Geometry: final body of the model. Coordinates: model frame, mm. Face numbers are marked on the shaded views. A direction names the side the tool comes from. Coordinates: 2 decimals unless noted, no trailing zeros. Write each loop counter-clockwise with the first axis right and the second up, starting at its lowest first coordinate (ties: lowest second). Pieces come first, ordered by that corner, then holes. Notation, with made-up numbers: (-7.5, -28) - (34.5, -28) arc R22 ccw to (34.5, -22) - close; hole circle Ø7 at (38, 38.5). An arc over 180 degrees is marked (long way). Put each result on its own line as item: value.
```python
from build123d import *

# Parameters (mm, degrees)
SCHIZZO1_R                   = 9.5
SCHIZZO1_R_2                 = 4.15
ESTRUSIONE_ESTRUSIONE1_DEPTH = 40
SCHIZZO2_W                   = 20.1
SCHIZZO2_H                   = 10.1
TAGLIO_ESTRUSIONE1_DEPTH     = 46.290727528
SMUSSO1_SIZE                 = 9
SMUSSO1_SIZE2                = 5
RACCORDO1_R                  = 1
SCHIZZO3_R                   = 6.125
TAGLIO_ESTRUSIONE2_DEPTH     = 35


with BuildPart() as part:
    # Schizzo1 → Estrusione-Estrusione1 (new body)
    with BuildSketch(Plane.XY):
        Circle(SCHIZZO1_R)
        Circle(SCHIZZO1_R_2, mode=Mode.SUBTRACT)
    extrude(amount=ESTRUSIONE_ESTRUSIONE1_DEPTH)

    # Schizzo2 → Taglio-Estrusione1 (cut, through all)
    with BuildSketch(Plane(origin=(9.5, 0, 0), x_dir=(0, 0, -1), z_dir=(1, 0, 0))):
        with Locations((-19.95, 0)):
            Rectangle(SCHIZZO2_W, SCHIZZO2_H)
    extrude(amount=-TAGLIO_ESTRUSIONE1_DEPTH, mode=Mode.SUBTRACT)

    # Smusso1
    smusso1_edges = [part.edges().sort_by_distance(p)[0] for p in [
        (-9.5, 0, 0),
        (-9.5, 0, 40),
    ]]
    smusso1_side = [part.faces().sort_by_distance(p)[0] for p in [
        (-9.5, 0, 20),
    ]]
    chamfer(smusso1_edges, length=SMUSSO1_SIZE, length2=SMUSSO1_SIZE2, reference=smusso1_side[0])

    # Raccordo1
    # the kernel refuses this fillet: 1 mm, written as the material it takes off along each edge
    with BuildSketch(Plane(origin=(0, 0, 40), x_dir=(1, 0, 0), z_dir=(0, -1, 0))) as raccordo1_piece_1:
        with BuildLine():
            CenterArc((3.892925278, -0.966391529), RACCORDO1_R, 29.054604099, 46.048838888)
            Line((4.15, 0), (4.155141494, 0.019327831))
            ThreePointArc((4.155141494, 0.019327831), (4.325, 0.02), (4.5, 0.02))
            Line((4.5, 0.02), (4.517483146, 0.009712859))
            Line((4.517483146, 0.009712859), (4.7845657, -0.471035739))
            Line((4.7845657, -0.471035739), (4.767082554, -0.480748598))
        make_face()
    revolve(axis=Axis((0, 0, 40), (0, 0, 1)), mode=Mode.SUBTRACT)

    # Schizzo3 → Taglio-Estrusione2 (cut)
    with BuildSketch(Plane(origin=(0, 0, 0), x_dir=(-1, 0, 0), z_dir=(0, 0, -1))):
        Circle(SCHIZZO3_R)
    extrude(amount=-TAGLIO_ESTRUSIONE2_DEPTH, mode=Mode.SUBTRACT)


solid = part.part
```
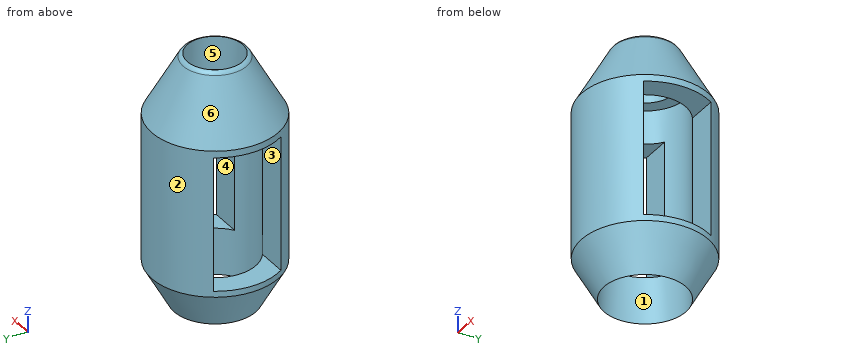
1. Section query A-A (y = 0). Return loops of the section in (x, z) (3 decimals), then the cut area to 3 significant figures.
Answer below:
outline: (-9.5, 9) - (-6.125, 2.925) - (-6.125, 9.9) - (-9.5, 9.9) - close; (-9.5, 30) - (-6.125, 30) - (-6.125, 35) - (-4.15, 35) - (-4.15, 40) arc R1 ccw to (-4.767, 39.519) - (-9.5, 31) - close; (4.15, 35) - (6.125, 35) - (6.125, 30) - (9.5, 30) - (9.5, 31) - (4.767, 39.519) arc R1 ccw to (4.15, 40) - close; (6.125, 2.925) - (9.5, 9) - (9.5, 9.9) - (6.125, 9.9) - close
area: 68.7 mm²
2. Section query C-C (x = 0). Return loops of the section in (y, z) (3 decimals).
Answer below:
outline: (-9.5, 9) - (-6.125, 2.925) - (-6.125, 35) - (-4.15, 35) - (-4.15, 40) arc R1 ccw to (-4.767, 39.519) - (-9.5, 31) - close; (4.15, 35) - (6.125, 35) - (6.125, 2.925) - (9.5, 9) - (9.5, 31) - (4.767, 39.519) arc R1 ccw to (4.15, 40) - close
3. Section query D-D (z = 9.5). Return loops of the section in (x, y) (3 decimals).
Answer below:
outline: circle Ø19 at (0, 0); hole circle Ø12.25 at (0, 0)
4. Pin query (flat end, axial travel): pin 1 Ø3 at (x, y) = (7.5, 2) entering from +Z; pin 2 Ø3.5 at (x, z) = (5.5, 21.5) entering from +Y; pin 3 Ø10 at (x, y) = (0, 0) entering from -Z. Return the tip coordinate at first contact, or that it passes through.
Answer below:
pin 1: stops at z = 36.83
pin 2: stops at y = 8.73
pin 3: stops at z = 35
5. Mould query, pull axis Z, two halves, no side actions, for the marked faces 4, 5 and 6. Classes: +Z half, -Z half, draft (parallel to the pull), parting line (faces both ways), or undercut.
Answer below:
face 4: undercut
face 5: draft
face 6: +Z half
6. Ray query, probe 1 along Y at (x, z) = (0, 26) (3 decimals); probe 2 along X at (y, z) = (-3.75, 38.5); probe 3 along Y at (x, z) = (5, 15.5). Return the intervals inside material, ascending. Write a range as from..to.
Answer below:
probe 1: y = -9.5..-6.125, 6.125..9.5
probe 2: x = -3.79..-1.78, 1.78..3.79
probe 3: y = -8.08..-5.05, 5.05..8.08
7. Section query B-B (z = 18). Return loops of the section in (x, y) (3 decimals).
Answer below:
outline: (-8.047, -5.05) arc R9.5 ccw to (8.047, -5.05) - (3.466, -5.05) arc R6.125 cw to (-3.466, -5.05) - close; (-8.047, 5.05) - (-3.466, 5.05) arc R6.125 cw to (3.466, 5.05) - (8.047, 5.05) arc R9.5 ccw to start
8. Set-up query: the marked faces 1, 2 and 3. Return all of +Z, -Z, +X, -X, +Y, -Y with unobstructed straight access to the full face (end or side cutting, diameter ignored); none if empty.
Answer below:
face 1: -Z
face 2: +Z, -Z
face 3: +X, -X
